Read the model definition and answer for the solid it produces. Units are mm, in the model's axes. Face numbers are marked on the shaded views. Coordinates: 2 decimals unless noted, no trailing zeros. Write each loop counter-clockwise with the first axis right and the second up, starting at its lowest first coordinate (ties: lowest second). Pieces come first, ordered by that corner, then holes. Notation, with made-up numbers: (34.5, -16.75) -> (46.5, -16.75) arc R19 cw to (46.5, 1.25) -> close; hole circle Ø7 at (-9, -38). An arc over 180 degrees is marked (long way). One line per item, written item: value. Start each with the question number.
1. Find section D-D, the plane y = -0.5. Write down the section's boundary in (x, z).
2. For a pull along Z with two mould halves and no side action, classify the marked faces 1 and 2 as pulls with the +Z half, pulls with the -Z half, needs draft (parallel to the pull), parting line crosses it, or undercut.
3. Find section A-A, the plane x = 0. Write down the section's boundary in (y, z).
4. Find section C-C, the plane y = -8.5. Write down the section's boundary in (x, z), and give its area (3 significant figures).
5. Find section B-B, the plane z = 0. Write down the section's boundary in (x, y).
6. Consider line 1 along Z through (x, y) = (0, -6.5); line 2 along Y through (x, z) = (-1.5, 8); line 3 along Z through (x, y) = (4, -4). Determine where each line is inside the solid, lowest interval first.
7. Given P1, Ø3, axis at y = 8.5, z = -7, coming from the +X side; P2, Ø8, axis at x = 5.5, y = 9, coming from the +Z side; P3, Ø6, axis at y = -19.5, z = -6, coming from the +X side; P4, Ø2, axis at x = 5, z = -0.5, coming from the +Y side, each flat-ended and moving along its own axis, determine where each tip first touches the part or whether it passes through.
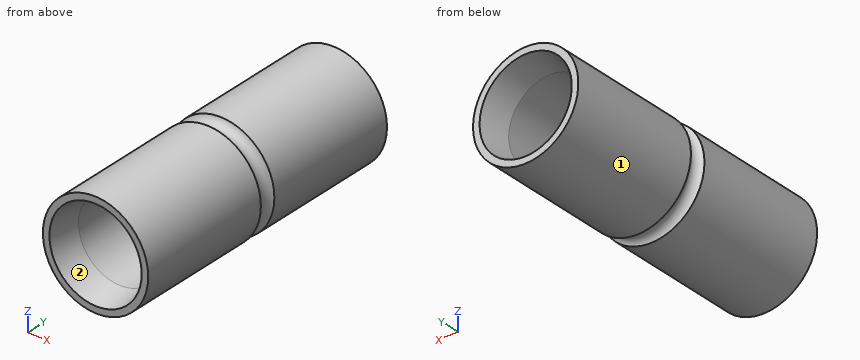
Solid Edge part; units mm, degrees
sketch "Sketch1" plane through (0, 0, 0) normal (0, -1, 0) x (1, 0, 0)
  circle A0 centre (0, 0) radius 9
  circle A1 centre (0, 0) radius 7
extrude "Protrusion1" add sketch "Sketch1" along normal mid plane 50
sketch "Sketch2" plane through (0, 0, 0) normal (0, 0, 1) x (1, 0, 0)
  circle A0 centre (-9.5, 0) radius 1.5
revolve "RevolvedCutout1" cut sketch "Sketch2" angle 360 about axis through (0, 54, 0) along (0, -1, 0)
chamfer "Chanfro_1" distance 5 angle 10 2 edges at (-7, -25, 0) (-7, 25, 0) measured on face at (3.8737, -20.5833, 5.8304) measured on face at (3.8737, 20.5833, 5.8304)
Answer block:
1. outline: circle Ø16.17 at (0, 0); hole circle Ø14 at (0, 0)
2. face 1: parting line crosses it
2. face 2: undercut
3. outline: (-25, -9) -> (-1.41, -9) arc R1.5 cw to (1.41, -9) -> (25, -9) -> (25, -7.88) -> (20, -7) -> (-20, -7) -> (-25, -7.88) -> close; (-25, 7.88) -> (-20, 7) -> (20, 7) -> (25, 7.88) -> (25, 9) -> (1.41, 9) arc R1.5 cw to (-1.41, 9) -> (-25, 9) -> close
4. outline: circle Ø18 at (0, 0); hole circle Ø14 at (0, 0)
4. area: 101 mm2
5. outline: (-9, -25) -> (-7.88, -25) -> (-7, -20) -> (-7, 20) -> (-7.88, 25) -> (-9, 25) -> (-9, 1.41) arc R1.5 cw to (-9, -1.41) -> close; (7, -20) -> (7.88, -25) -> (9, -25) -> (9, -1.41) arc R1.5 cw to (9, 1.41) -> (9, 25) -> (7.88, 25) -> (7, 20) -> close
6. line 1: z = -9 to -7, 7 to 9
6. line 2: y = -25 to -0.63, 0.63 to 25
6. line 3: z = -8.06 to -5.74, 5.74 to 8.06
7. P1: stops at x = 7.12
7. P2: stops at z = 8.87
7. P3: stops at x = 8.49
7. P4: passes through
